Input: part model. Units: mm. Frame: model coordinates. Round coordinates to 2 decimals unless told otherwise and drop trailing zeros. Use a Markdown table: item, result.
from build123d import *

# Parameters (mm, degrees)
SKETCH003_R         = 2.1
PAD003_DEPTH        = 490
CHAMFER003_1_ANGLE  = 45
CHAMFER003_1_SIZE   = 1.7
CHAMFER003_2_ANGLE  = 45
CHAMFER003_2_SIZE   = 1.7
CHAMFER003_3_ANGLE  = 45
CHAMFER003_3_SIZE   = 1.7
CHAMFER003_4_ANGLE  = 45
CHAMFER003_4_SIZE   = 1.7
CHAMFER003_5_ANGLE  = 45
CHAMFER003_5_SIZE   = 1.7
CHAMFER003_6_ANGLE  = 45
CHAMFER003_6_SIZE   = 1.7
CHAMFER003_7_ANGLE  = 45
CHAMFER003_7_SIZE   = 1.7
CHAMFER003_8_ANGLE  = 45
CHAMFER003_8_SIZE   = 1.7
CHAMFER003_9_ANGLE  = 45
CHAMFER003_9_SIZE   = 1.7
CHAMFER003_10_ANGLE = 45
CHAMFER003_10_SIZE  = 1.7
CHAMFER003_11_ANGLE = 45
CHAMFER003_11_SIZE  = 1.7
CHAMFER003_12_ANGLE = 45
CHAMFER003_12_SIZE  = 1.7
FILLET003_R         = 0.2


with BuildPart() as part:
    # Sketch003 → Pad003 (new body)
    with BuildSketch(Plane.XY):
        Polygon((0, 3.723883), (0.176777, 3.90066), (2.84, 3.90066), (5.49934, 6.56), (5.49934, 8.2), (3.1, 8.2), (3.1, 10), (16.9, 10), (16.9, 8.2), (14.50066, 8.2), (14.50066, 6.56), (17.16, 3.90066), (19.823223, 3.90066), (20, 3.723883), (20.176777, 3.90066), (22.84, 3.90066), (25.49934, 6.56), (25.49934, 8.2), (23.1, 8.2), (23.1, 10), (30, 10), (30, 3.1), (28.2, 3.1), (28.2, 5.49934), (26.56, 5.49934), (23.90066, 2.84), (23.90066, 0.176777), (23.723883, 0), (23.90066, -0.176777), (23.90066, -2.84), (26.56, -5.49934), (28.2, -5.49934), (28.2, -3.1), (30, -3.1), (30, -10), (23.1, -10), (23.1, -8.2), (25.49934, -8.2), (25.49934, -6.56), (22.84, -3.90066), (20.176777, -3.90066), (20, -3.723883), (19.823223, -3.90066), (17.16, -3.90066), (14.50066, -6.56), (14.50066, -8.2), (16.9, -8.2), (16.9, -10), (3.1, -10), (3.1, -8.2), (5.49934, -8.2), (5.49934, -6.56), (2.84, -3.90066), (0.176777, -3.90066), (0, -3.723883), (-0.176777, -3.90066), (-2.84, -3.90066), (-5.49934, -6.56), (-5.49934, -8.2), (-3.1, -8.2), (-3.1, -10), (-10, -10), (-10, -3.1), (-8.2, -3.1), (-8.2, -5.49934), (-6.56, -5.49934), (-3.90066, -2.84), (-3.90066, -0.176777), (-3.723883, 0), (-3.90066, 0.176777), (-3.90066, 2.84), (-6.56, 5.49934), (-8.2, 5.49934), (-8.2, 3.1), (-10, 3.1), (-10, 10), (-3.1, 10), (-3.1, 8.2), (-5.49934, 8.2), (-5.49934, 6.56), (-2.84, 3.90066), (-0.176777, 3.90066), align=None)
        Circle(SKETCH003_R, mode=Mode.SUBTRACT)
        with Locations((20, 0)):
            Circle(SKETCH003_R, mode=Mode.SUBTRACT)
        Polygon((7.29934, 6.23868), (3.90066, 2.84), (3.90066, 0.176777), (3.723883, 0), (3.90066, -0.176777), (3.90066, -2.84), (7.29934, -6.23868), (7.29934, -8.2), (12.70066, -8.2), (12.70066, -6.23868), (16.09934, -2.84), (16.09934, -0.176777), (16.276117, 0), (16.09934, 0.176777), (16.09934, 2.84), (12.70066, 6.23868), (12.70066, 8.2), (7.29934, 8.2), align=None, mode=Mode.SUBTRACT)
    extrude(amount=PAD003_DEPTH)

    # Chamfer003 1
    chamfer003_1_edges = [part.edges().sort_by_distance(p)[0] for p in [
        (3.1, -10, 245),
    ]]
    chamfer003_1_side = part.faces().sort_by_distance((10, -10, 245))[0]
    chamfer(chamfer003_1_edges, length=CHAMFER003_1_SIZE, angle=CHAMFER003_1_ANGLE, reference=chamfer003_1_side)

    # Chamfer003 2
    chamfer003_2_edges = [part.edges().sort_by_distance(p)[0] for p in [
        (16.9, -10, 245),
    ]]
    chamfer003_2_side = part.faces().sort_by_distance((16.9, -9.1, 245))[0]
    chamfer(chamfer003_2_edges, length=CHAMFER003_2_SIZE, angle=CHAMFER003_2_ANGLE, reference=chamfer003_2_side)

    # Chamfer003 3
    chamfer003_3_edges = [part.edges().sort_by_distance(p)[0] for p in [
        (23.1, -10, 245),
    ]]
    chamfer003_3_side = part.faces().sort_by_distance((26.55, -10, 245))[0]
    chamfer(chamfer003_3_edges, length=CHAMFER003_3_SIZE, angle=CHAMFER003_3_ANGLE, reference=chamfer003_3_side)

    # Chamfer003 4
    chamfer003_4_edges = [part.edges().sort_by_distance(p)[0] for p in [
        (-3.1, -10, 245),
    ]]
    chamfer003_4_side = part.faces().sort_by_distance((-3.1, -9.1, 245))[0]
    chamfer(chamfer003_4_edges, length=CHAMFER003_4_SIZE, angle=CHAMFER003_4_ANGLE, reference=chamfer003_4_side)

    # Chamfer003 5
    chamfer003_5_edges = [part.edges().sort_by_distance(p)[0] for p in [
        (30, -3.1, 245),
    ]]
    chamfer003_5_side = part.faces().sort_by_distance((29.1, -3.1, 245))[0]
    chamfer(chamfer003_5_edges, length=CHAMFER003_5_SIZE, angle=CHAMFER003_5_ANGLE, reference=chamfer003_5_side)

    # Chamfer003 6
    chamfer003_6_edges = [part.edges().sort_by_distance(p)[0] for p in [
        (30, 3.1, 245),
    ]]
    chamfer003_6_side = part.faces().sort_by_distance((30, 6.55, 245))[0]
    chamfer(chamfer003_6_edges, length=CHAMFER003_6_SIZE, angle=CHAMFER003_6_ANGLE, reference=chamfer003_6_side)

    # Chamfer003 7
    chamfer003_7_edges = [part.edges().sort_by_distance(p)[0] for p in [
        (23.1, 10, 245),
    ]]
    chamfer003_7_side = part.faces().sort_by_distance((23.1, 9.1, 245))[0]
    chamfer(chamfer003_7_edges, length=CHAMFER003_7_SIZE, angle=CHAMFER003_7_ANGLE, reference=chamfer003_7_side)

    # Chamfer003 8
    chamfer003_8_edges = [part.edges().sort_by_distance(p)[0] for p in [
        (16.9, 10, 245),
    ]]
    chamfer003_8_side = part.faces().sort_by_distance((10, 10, 245))[0]
    chamfer(chamfer003_8_edges, length=CHAMFER003_8_SIZE, angle=CHAMFER003_8_ANGLE, reference=chamfer003_8_side)

    # Chamfer003 9
    chamfer003_9_edges = [part.edges().sort_by_distance(p)[0] for p in [
        (3.1, 10, 245),
    ]]
    chamfer003_9_side = part.faces().sort_by_distance((3.1, 9.1, 245))[0]
    chamfer(chamfer003_9_edges, length=CHAMFER003_9_SIZE, angle=CHAMFER003_9_ANGLE, reference=chamfer003_9_side)

    # Chamfer003 10
    chamfer003_10_edges = [part.edges().sort_by_distance(p)[0] for p in [
        (-3.1, 10, 245),
    ]]
    chamfer003_10_side = part.faces().sort_by_distance((-6.55, 10, 245))[0]
    chamfer(chamfer003_10_edges, length=CHAMFER003_10_SIZE, angle=CHAMFER003_10_ANGLE, reference=chamfer003_10_side)

    # Chamfer003 11
    chamfer003_11_edges = [part.edges().sort_by_distance(p)[0] for p in [
        (-10, -3.1, 245),
    ]]
    chamfer003_11_side = part.faces().sort_by_distance((-10, -6.55, 245))[0]
    chamfer(chamfer003_11_edges, length=CHAMFER003_11_SIZE, angle=CHAMFER003_11_ANGLE, reference=chamfer003_11_side)

    # Chamfer003 12
    chamfer003_12_edges = [part.edges().sort_by_distance(p)[0] for p in [
        (-10, 3.1, 245),
    ]]
    chamfer003_12_side = part.faces().sort_by_distance((-9.1, 3.1, 245))[0]
    chamfer(chamfer003_12_edges, length=CHAMFER003_12_SIZE, angle=CHAMFER003_12_ANGLE, reference=chamfer003_12_side)

    # Fillet003
    fillet003_edges = [part.edges().sort_by_distance(p)[0] for p in [
        (-10, -10, 245),
        (-10, 10, 245),
        (30, 10, 245),
        (30, -10, 245),
    ]]
    fillet(fillet003_edges, radius=FILLET003_R)


solid = part.part
1) Cut plane A-A on z = 281. State how many separate pieces and enclosed holes the cut face has, and give its area (3 significant figures).
Answer key:
| item | result |
|---|---|
| separate pieces | 1 |
| enclosed holes | 3 |
| area | 296 mm^2 |
2) Ray query, probe 1 along X at (y, z) = (7.75, 385.5); probe 2 along Y at (x, z) = (20, 347); probe 3 along X at (y, z) = (-8.5, 278.5). Return the intervals inside material, ascending.
Answer key:
| item | result |
|---|---|
| probe 1 | x = -10 to -5.5, 5.5 to 7.3, 12.7 to 14.5, 25.5 to 30 |
| probe 2 | y = -3.72 to -2.1, 2.1 to 3.72 |
| probe 3 | x = -10 to -3.3, 3.3 to 16.7, 23.3 to 30 |
3) Contact query for flat-ended pins moving along their axis: P1, Ø1.3, axis at x = 18.5, z = 296.5, coming from the -Y side; P2, Ø2, axis at x = -1, z = 348.5, coming from the +Y side; P3, Ø1.2, axis at y = -4, z = 287, coming from the +X side; P4, Ø1.5, axis at x = 20, y = -6, coming from the +Z side. Output: stop coordinate, or through.
Answer key:
| item | result |
|---|---|
| P1 | stops at y = -3.9 |
| P2 | stops at y = 3.9 |
| P3 | stops at x = 29.8 |
| P4 | passes through |
